from build123d import *

# Parameters (mm, degrees)
SKICA2_OUTSIDE_W              = 119.114
SKICA2_OUTSIDE_H              = 64.114
SKICA2_OUTSIDE_W_2            = 160.751096763
SKICA2_OUTSIDE_H_2            = 21.9
ODEBRAT_VYSUNUT_M1_DEPTH      = 21
ODEBRAT_VYSUNUT_M1_DEPTH_BACK = 21
SKICA3_R                      = 10
ODEBRAT_VYSUNUT_M2_DEPTH      = 11.95
ODEBRAT_VYSUNUT_M2_DEPTH_BACK = 11.95
ZKOSEN_1_SIZE                 = 1
ZKOSEN_2_SIZE                 = 2


with BuildPart() as part:
    # Skica1 → Rotovat1 (revolve)
    with BuildSketch(Plane.XY, mode=Mode.PRIVATE) as rotovat1_sk:
        with BuildLine():
            Line((7.101020514, 18.696938457), (30, 10))
            Line((30, 10), (75, 10))
            Line((75, 10), (75, 0))
            Line((75, 0), (-20, 0))
            ThreePointArc((-20, 0), (-11.357367426, 16.462387589), (7.101020514, 18.696938457))
        make_face()
    revolve(rotovat1_sk.sketch.rotate(Axis((0, 0, 0), (-1, 0, 0)), 90), axis=Axis((0, 0, 0), (-1, 0, 0)))  # turned: the seam where the file's is

    # Skica2 outside → Odebrat vysunutím1 (cut, two sides)
    with BuildSketch(Plane(origin=(0, 0, 0), x_dir=(1, 0, 0), z_dir=(0, 1, 0))) as odebrat_vysunut_m1_sk:
        with Locations((27.5, 0)):
            Rectangle(SKICA2_OUTSIDE_W, SKICA2_OUTSIDE_H)
        with Locations((14.564667135, 0)):
            Rectangle(SKICA2_OUTSIDE_W_2, SKICA2_OUTSIDE_H_2, mode=Mode.SUBTRACT)
    extrude(amount=ODEBRAT_VYSUNUT_M1_DEPTH, mode=Mode.SUBTRACT)
    extrude(odebrat_vysunut_m1_sk.sketch, amount=-ODEBRAT_VYSUNUT_M1_DEPTH_BACK, mode=Mode.SUBTRACT)

    # Skica3 → Odebrat vysunutím2 (cut, two sides)
    with BuildSketch(Plane.XY) as odebrat_vysunut_m2_sk:
        Circle(SKICA3_R)
    extrude(amount=ODEBRAT_VYSUNUT_M2_DEPTH, mode=Mode.SUBTRACT)
    extrude(odebrat_vysunut_m2_sk.sketch, amount=-ODEBRAT_VYSUNUT_M2_DEPTH_BACK, mode=Mode.SUBTRACT)

    # Zkosení1
    zkosen_1_edges = [part.edges().sort_by_distance(p)[0] for p in [
        (-10, 0, -10.95),
        (-10, 0, 10.95),
    ]]
    chamfer(zkosen_1_edges, length=ZKOSEN_1_SIZE)

    # Zkosení2
    zkosen_2_edges = [part.edges().sort_by_distance(p)[0] for p in [
        (75, 0, 10),
    ]]
    chamfer(zkosen_2_edges, length=ZKOSEN_2_SIZE)


solid = part.part
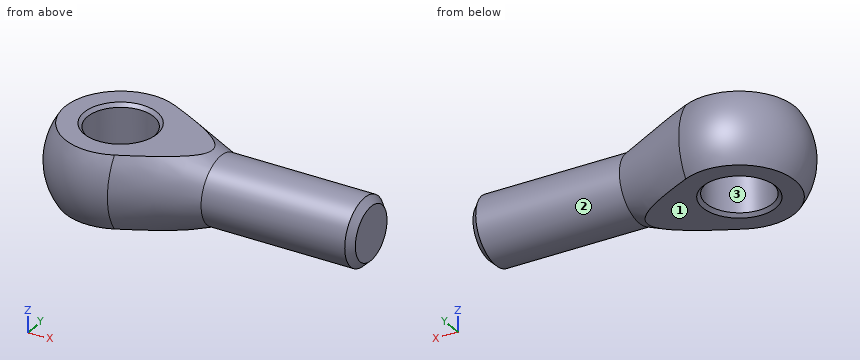
The model under review builds one solid part; all positions refer to its coordinate system, in mm. Face numbers are marked on the shaded views. Give positions to 0.01 mm unless a question says otherwise; leave off trailing zeros. Order: outer loops, then holes, each group sorted by start corner. A loop starts at its lowest first (then second) coordinate and runs counter-clockwise, first axis right, second up. Notation, with made-up numbers: M 40.5,49.25 L 70.5,49.25 A21 ccw 70.5,85.25 Z; hole C 55.5,-21 d5. An arc over 180 degrees is marked long. One line per question, with ' | ' between items. Start each with the question number.
1) Consider section C-C, the plane z = 0. Give the boundary of the cut face in (x, y).
2) Clearance check with flat-ended pins moving along their axes: P1, Ø3, axis at x = 44.5, z = 2, coming from the +Y side; P2, Ø3, axis at x = 60.5, z = 5, coming from the +Y side; P3, Ø10, axis at x = 27.5, y = 9.5, coming from the -Z side. State where each tip first meets the part, or that it passes through.
3) Consider section D-D, the plane x = 63. Give the boundary of the cut face in (y, z), then the cut area to 3 significant figures.
4) Wall thickness on L1, parallel to X at y = 0, z = 0.5; L2, parallel to X at y = 0, z = 5.75; L3, parallel to Y at x = -1.5, z = -4: over which ranges is each line inside the solid? List them lowest first. Write a range as from..to.
5) Consider section B-B, the plane y = 0. Give the boundary of the cut face in (x, z), then the cut area to 3 significant figures.
6) Consider section A-A, the plane x = 0. Give the boundary of the cut face in (y, z).
7) Mouldability with a two-part tool opening along Y and no side actions: class the marked faces 1, 2 and 3 as pulls with the +Y half, pulls with the -Y half, needs draft (parallel to the pull), parting line crosses it, or undercut.
Found:
1) outline: M 7.1,-18.7 L 30,-10 L 73,-10 L 75,-8 L 75,8 L 73,10 L 30,10 L 7.1,18.7 A20 ccw long Z; hole C 0,0 d20
2) P1: stops at y = 9.99 | P2: stops at y = 9.37 | P3: stops at z = -10.77
3) outline: C 0,0 d20 | area: 314 mm²
4) L1: x = -19.99..-10, 10..75 | L2: x = -19.16..-10, 10..75 | L3: y = -19.54..-9.89, 9.89..19.54
5) outline: M -16.74,-10.95 L -11,-10.95 L -10,-9.95 L -10,9.95 L -11,10.95 L -16.74,10.95 A20 ccw Z; M 10,-9.95 L 11,-10.95 L 27.5,-10.95 L 30,-10 L 73,-10 L 75,-8 L 75,8 L 73,10 L 30,10 L 27.5,10.95 L 11,10.95 L 10,9.95 Z | area: 1,530 mm²
6) outline: M -16.74,-10.95 L -11,-10.95 L -10,-9.95 L -10,9.95 L -11,10.95 L -16.74,10.95 A20 ccw Z; M 10,-9.95 L 11,-10.95 L 16.74,-10.95 A20 ccw 16.74,10.95 L 11,10.95 L 10,9.95 Z
7) face 1: needs draft | face 2: parting line crosses it | face 3: undercut
